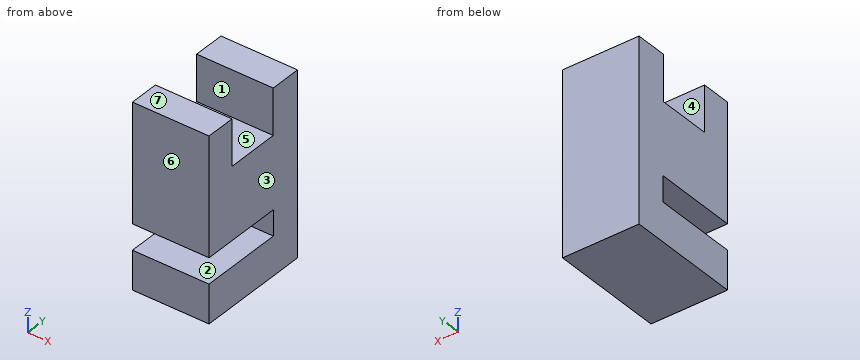
```python
from build123d import *

# Parameters (mm, degrees)
F1_DEPTH = 10
F2_W     = 10
F2_H     = 4.121232
F2_H_2   = 3.88832
F3_DEPTH = 6


with BuildPart() as f1:
    # F0 (on Right) → F1 (new body)
    with BuildSketch(Plane.YZ):
        Polygon((-15.009552, 0), (0, 0), (0, 17.770922), (-15.009552, 17.770922), (-15.009552, 8.370922), (-4.10229, 8.370922), (-4.10229, 5.044594), (-15.009552, 5.044594), align=None)
    extrude(amount=F1_DEPTH)

    # F2 (on face) → F3 (join)
    with BuildSketch(Plane.XY.offset(17.770922)):
        with Locations((5, -2.060616)):
            Rectangle(F2_W, F2_H)
        with Locations((5, -13.065392)):
            Rectangle(F2_W, F2_H_2)
    extrude(amount=F3_DEPTH)


solid = f1.part
```
Model file for the job. Use its own axes, mm. Face numbers are marked on the shaded views. A direction names the side the tool comes from. Give positions to 0.01 mm unless a question says otherwise; leave off trailing zeros. Loops run counter-clockwise (first coordinate to the right, second up) from the corner with the lowest first, then second, coordinate; pieces in that order, holes last. Notation, with made-up numbers: (51, 59.25) -> (56, 59.25) arc R8 cw to (56, 63.25) -> close; hole circle Ø6 at (36, 29). An arc over 180 degrees is marked (long way). Use CSV: the item, a comma, the result in double quotes. Start each with the question number.
1) Slice it at B-B on x = 4.5. Give the cut face in (y, z).
2) Tool access for the marked faces 1, 2 and 3: list every direction of +Z, -Z, +X, -X, +Y, -Y with a clear straight run to the whole face (end or side of a thin tool).
3) Flat gauge pins, fed straight in: pin 1 Ø4 at (x, z) = (5, 7.5) entering from -Y; pin 2 Ø3.5 at (x, y) = (3.5, -7.5) entering from +Z. Where does each tip first touch, or does it go through?
4) Mould opens along Y. For the marked faces 4, 5, 6 and 7 say: released by +Y, released by -Y, zero draft, split by the parting line, or undercut.
5) Slice it at A-A on y = -7.25. Give the cut face in (x, z), plus the area to 3 significant figures.
6) Wall check: line 1 (Y direction, x = 1.5, z = 21); line 2 (Z direction, x = 6.75, y = -7.5); line 3 (Z direction, x = 9, y = -12.5). Give the ranges that are in metal, low to high.
Computed values:
1,outline,"(-15.01, 0) -> (0, 0) -> (0, 23.77) -> (-4.12, 23.77) -> (-4.12, 17.77) -> (-11.12, 17.77) -> (-11.12, 23.77) -> (-15.01, 23.77) -> (-15.01, 8.37) -> (-4.1, 8.37) -> (-4.1, 5.04) -> (-15.01, 5.04) -> close"
2,face 1,"+Z, +X, -X"
2,face 2,"+X, -X, -Y"
2,face 3,"+Z, -Z, +X, +Y, -Y"
3,pin 1,"stops at y = -15.01"
3,pin 2,"stops at z = 17.77"
4,face 4,"undercut"
4,face 5,"undercut"
4,face 6,"released by -Y"
4,face 7,"zero draft"
5,outline,"(0, 0) -> (10, 0) -> (10, 5.04) -> (0, 5.04) -> close; (0, 8.37) -> (10, 8.37) -> (10, 17.77) -> (0, 17.77) -> close"
5,area,"144 mm^2"
6,line 1,"y = -15.01 to -11.12, -4.12 to 0"
6,line 2,"z = 0 to 5.04, 8.37 to 17.77"
6,line 3,"z = 0 to 5.04, 8.37 to 23.77"
